```python
from build123d import *

# Parameters (mm, degrees)
BOSS_EXTRUDE1_DEPTH     = 10
BOSS_EXTRUDE1_2_DEPTH   = 10
BOSS_EXTRUDE1_3_DEPTH   = 10
BOSS_EXTRUDE5_DEPTH     = 55
SKETCH5_W               = 18.5
SKETCH5_H               = 5.5
BOSS_EXTRUDE6_DEPTH     = 8
SKETCH6_W               = 18.5
SKETCH6_H               = 5.5
BOSS_EXTRUDE7_DEPTH     = 8
BOSS_EXTRUDE8_OUTLINE_W = 18.287900599
BOSS_EXTRUDE8_OUTLINE_H = 18.500510452
BOSS_EXTRUDE8_DEPTH     = 14
SKETCH7_3_R             = 2.25
CUT_EXTRUDE1_DEPTH      = 10


# Read off the part's stored shape, not the designer's step: Boss-Extrude8
with BuildPart() as part:
    # Sketch1 → Boss-Extrude1 (new body)
    with BuildSketch(Plane(origin=(0, 0, 0), x_dir=(1, 0, 0), z_dir=(0, 1, 0))):
        Polygon((-54.711603102, -80), (-54.711603102, -28.907893648), (-27.826820773, -10.273471277), (-46.326820773, -10.048678982), (-46.460237213, 8.450839932), (-27.961603102, 8.226037736), (-54.711603102, 28.907893648), (-54.711603102, 80), (-73.211603102, 80), (-73.211603102, -80), align=None)
    extrude(amount=BOSS_EXTRUDE1_DEPTH)



with BuildPart() as body_2:
    # Sketch1 → Boss-Extrude1 2 (new body)
    with BuildSketch(Plane(origin=(0, 0, 0), x_dir=(1, 0, 0), z_dir=(0, 1, 0))):
        Polygon((-27.961603102, 8.226037736), (-27.826820773, -10.273471277), (28.173179227, -10.273471277), (27.961603102, 8.225318833), align=None)
    extrude(amount=BOSS_EXTRUDE1_2_DEPTH)


with BuildPart() as body_3:
    # Sketch1 → Boss-Extrude1 3 (new body)
    with BuildSketch(Plane(origin=(0, 0, 0), x_dir=(1, 0, 0), z_dir=(0, 1, 0))):
        Polygon((46.674397065, -10.272954842), (28.173179227, -10.273471277), (54.711603102, -28.907893648), (54.711603102, -80), (73.211603102, -80), (73.211603102, 80), (54.711603102, 80), (54.711603102, 28.907893648), (27.961603102, 8.225318833), (46.461603021, 8.227045158), align=None)
    extrude(amount=BOSS_EXTRUDE1_3_DEPTH)


with BuildPart() as part_1:
    add(part.part)

    add(body_2.part)  # Boss-Extrude5 merges body 2

    add(body_3.part)  # Boss-Extrude5 merges body 3
    # Sketch1<9> → Boss-Extrude5 (add)
    with BuildSketch(Plane(origin=(0, 0, 0), x_dir=(1, 0, 0), z_dir=(0, 1, 0))):
        Polygon((46.461603021, 8.227045158), (46.674397065, -10.272954842), (28.173179227, -10.273471277), (27.961603102, 8.225318833), align=None)
        Polygon((-27.961603102, 8.226037736), (-46.460237213, 8.450839932), (-46.326820773, -10.048678982), (-27.826820773, -10.273471277), align=None)
    extrude(amount=BOSS_EXTRUDE5_DEPTH)

    # Sketch5 → Boss-Extrude6 (add)
    with BuildSketch(Plane(origin=(28.052008971, 0, -0.32083911), x_dir=(0.011436547294728296, 0, 0.999934600554444), z_dir=(-0.999934600554444, 0, 0.011436547294728296))):
        with Locations((1.345003295, 52.25)):
            Rectangle(SKETCH5_W, SKETCH5_H)
    extrude(amount=BOSS_EXTRUDE6_DEPTH)

    # Sketch6 → Boss-Extrude7 (add)
    with BuildSketch(Plane(origin=(-27.900189464, 0, 0.203273098), x_dir=(-0.007285531290396893, 0, -0.9999734601647269), z_dir=(0.9999734601647269, 0, -0.007285531290396893))):
        with Locations((-0.820465448, 52.25)):
            Rectangle(SKETCH6_W, SKETCH6_H)
    extrude(amount=BOSS_EXTRUDE7_DEPTH)

    # Boss-Extrude8 outline → Boss-Extrude8 (add)
    with BuildSketch(Plane(origin=(0, 55, 0), x_dir=(1, 0, 0), z_dir=(0, 1, 0))):
        with Locations((-37.144162619, -1.023210068)):
            Rectangle(BOSS_EXTRUDE8_OUTLINE_W, BOSS_EXTRUDE8_OUTLINE_H)
        Polygon((46.461603021, -10.272960782), (46.461603021, 8.227045158), (28.173702422, 8.225338625), (28.173702422, -10.273471263), align=None)
    extrude(amount=BOSS_EXTRUDE8_DEPTH)

    # Sketch7<3> → Cut-Extrude1 (cut, symmetric)
    with BuildSketch(Plane(origin=(0, 55, 0), x_dir=(1, 0, 0), z_dir=(0, 1, 0))):
        with Locations(Location((24.147255407, 3.611254336, 0), (0, 0, 270))):
            Circle(SKETCH7_3_R)
        with Locations(Location((24.147255407, -5.842391538, 0), (0, 0, 270))):
            Circle(SKETCH7_3_R)
        with Locations(Location((-23.973765303, -5.842391538, 0), (0, 0, 270))):
            Circle(SKETCH7_3_R)
        with Locations(Location((-23.973765303, 3.611254336, 0), (0, 0, 270))):
            Circle(SKETCH7_3_R)
    extrude(amount=CUT_EXTRUDE1_DEPTH, both=True, mode=Mode.SUBTRACT)


solid = part_1.part
```
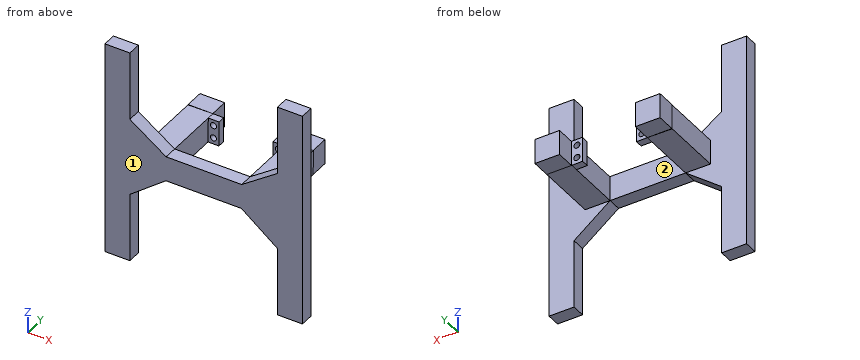
Work out the finished part from the listing and answer in its coordinate system (mm). Face numbers are marked on the shaded views. Coordinates: 2 decimals unless noted, no trailing zeros. Write each loop counter-clockwise with the first axis right and the second up, starting at its lowest first coordinate (ties: lowest second). Pieces come first, ordered by that corner, then holes. Notation, with made-up numbers: (16, -38) - (69, -38) arc R26 ccw to (69, -5) - close; hole circle Ø11 at (70, -36.5). An arc over 180 degrees is marked (long way). Answer as a JSON object with one key per item and string values.
Q1. Find section A-A (y = 63.5). Write down the section's boundary in (x, z).
Results list:
{"outline": "(-46.29, -8.23) - (-28, -8.23) - (-28, 10.27) - (-46.29, 10.27) - close; (28.17, -8.23) - (46.46, -8.23) - (46.46, 10.27) - (28.17, 10.27) - close"}
Q2. For a pull along X with two mould halves and no side action, classify the marked faces 1 and 2 as pulls with the +X half, pulls with the -X half, needs draft (parallel to the pull), parting line crosses it, or undercut.
Results list:
{"face 1": "needs draft", "face 2": "undercut"}
Q3. Find section B-B (z = 62). Write down the section's boundary in (x, y), plus the area to 3 significant figures.
Results list:
{"outline": "(-73.21, 0) - (-54.71, 0) - (-54.71, 10) - (-73.21, 10) - close; (54.71, 0) - (73.21, 0) - (73.21, 10) - (54.71, 10) - close", "area": "370 mm^2"}
Q4. Find section D-D (x = 38.5). Write down the section's boundary in (y, z), plus the area to 3 significant figures.
Results list:
{"outline": "(0, -16.37) - (10, -16.37) - (10, -8.23) - (69, -8.23) - (69, 10.27) - (10, 10.27) - (10, 17.52) - (0, 17.52) - close", "area": "1,430 mm^2"}
Q5. Given pin 1 Ø13.5 at (x, z) = (-41, 21) entering from +Y; pin 2 Ø7 at (x, y) = (39.5, 59) entering from -Z; pin 3 Ø11 at (y, z) = (63.5, 1) entering from -X, each flat-ended and moving along its own axis, determine where each tip first touches the part or whether it passes through.
Results list:
{"pin 1": "stops at y = 10", "pin 2": "stops at z = -8.23", "pin 3": "stops at x = -46.29"}
Q6. Find section C-C (y = 52). Write down the section's boundary in (x, z), plus the area to 3 significant figures.
Results list:
{"outline": "(-46.46, -8.45) - (-27.96, -8.23) - (-19.96, -8.28) - (-19.83, 10.22) - (-27.83, 10.27) - (-46.33, 10.05) - close; (19.96, -8.13) - (27.96, -8.23) - (46.46, -8.23) - (46.67, 10.27) - (28.17, 10.27) - (20.17, 10.36) - close; hole circle Ø4.5 at (-23.97, -3.61); hole circle Ø4.5 at (-23.97, 5.84); hole circle Ø4.5 at (24.15, -3.61); hole circle Ø4.5 at (24.15, 5.84)", "area": "917 mm^2"}
Q7. Consider L1, parallel to X at y = 9.5, z = -65; L2, parallel to X at y = 52.5, z = -5.5; L3, parallel to Y at x = 64.5, z = -73. Determine where each line is inside the solid, lowest interval first. Write a range as from..to.
Results list:
{"L1": "x = -73.21..-54.71, 54.71..73.21", "L2": "x = -46.44..-25.2, -22.75..-19.94, 19.99..22.92, 25.37..46.49", "L3": "y = 0..10"}
